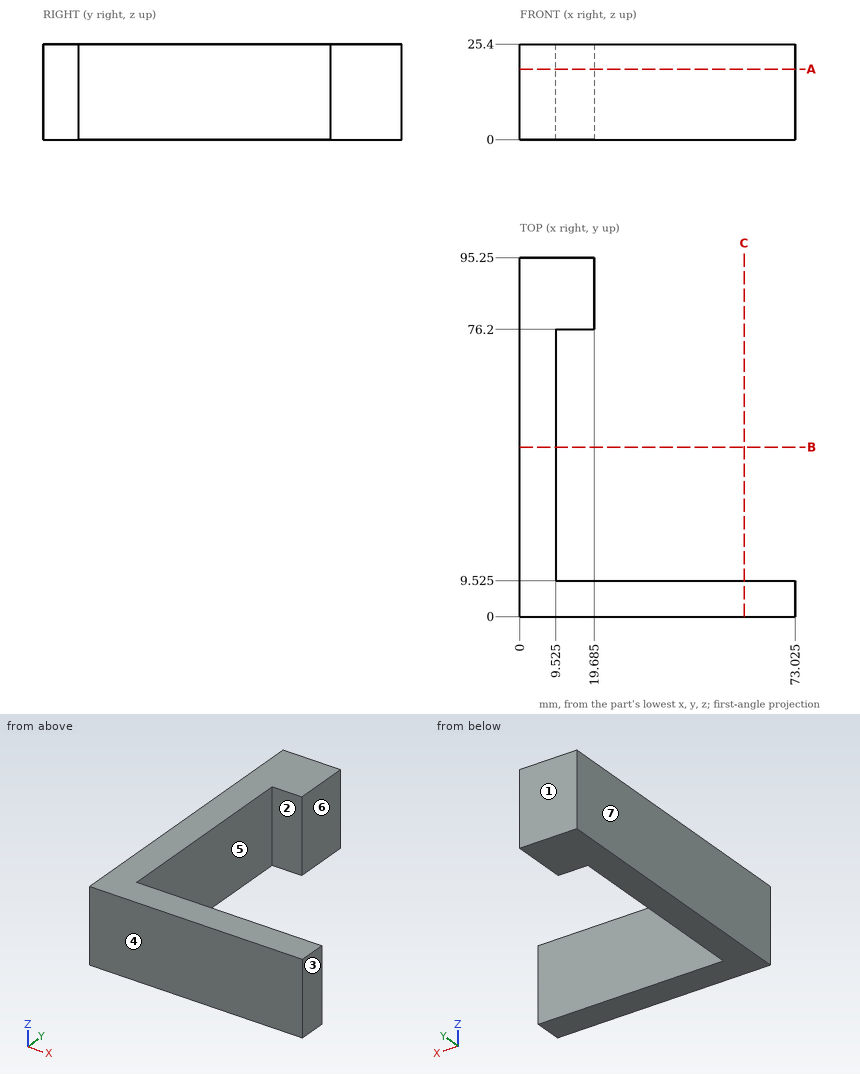
The figure shows three views and two pictorial views of one solid part (mm, origin at its lowest corner). Answer the questions. A direction names the side the tool comes from. Give positions to 0.01 mm unless a question says otherwise; leave off trailing zeros. Loops run counter-clockwise (first coordinate to the right, second up) from the corner with the lowest first, then second, coordinate; pieces in that order, holes last. Notation, with made-up numbers: (72.5, -38.5) -> (94.5, -38.5) arc R30 ccw to (94.5, -16.5) -> close; hole circle Ø6 at (56, 71). An arc over 180 degrees is marked (long way). Put each result on its own line as item: value. Start each with the question number.
Item 1: Find the intervals of material crossed by L1, parallel to Y at x = 13, z = 9.25 (3 decimals); L2, parallel to Y at x = 28.5, z = 13.25 (3 decimals), in increasing order. Write a range as [from, to].
Item 2: The part is cut by section B-B (y = 45). Give the vertices of the cut face in (x, z) (3 decimals), then the cut area to 3 significant figures.
Item 3: The mould has two halves that part along Y. Classify the marked faces 1, 2, 3 and 4: released by +Y, released by -Y, zero draft, split by the parting line, or undercut.
Item 4: Each of these flat-tipped pins is pushed along its axis until it touches: P1, Ø3, axis at y = 12, z = 10.5, coming from the +X side (3 decimals); P2, Ø10, axis at x = 58.5, z = 16.5, coming from the +Y side (3 decimals); P3, Ø5.5, axis at y = 89.5, z = 11, coming from the +X side (3 decimals). Where does it stop, or does it pass through?
Item 5: The part is cut by section A-A (z = 18.75). Give the vertices of the cut face in (x, y) (3 decimals), then the cut area to 3 significant figures.
Item 6: Which of the six approach directions +Z, -Z, +X, -X, +Y, -Y give full straight-line access (tool end or side, diameter ignored) to the marked faces 5, 6 and 7?
Answers below:
1. L1: [0, 9.525], [76.2, 95.25]
1. L2: [0, 9.525]
2. outline: (0, 0) -> (9.525, 0) -> (9.525, 25.4) -> (0, 25.4) -> close
2. area: 242 mm2
3. face 1: released by +Y
3. face 2: undercut
3. face 3: zero draft
3. face 4: released by -Y
4. P1: x = 9.525
4. P2: y = 9.525
4. P3: x = 19.685
5. outline: (0, 0) -> (73.025, 0) -> (73.025, 9.525) -> (9.525, 9.525) -> (9.525, 76.2) -> (19.685, 76.2) -> (19.685, 95.25) -> (0, 95.25) -> close
5. area: 1,710 mm2
6. face 5: +Z, -Z, +X
6. face 6: +Z, -Z, +X, +Y
6. face 7: +Z, -Z, -X, +Y, -Y
